Check sheet for the modelled part. Datum: model origin and axes. Units: mm. A direction names the side the tool comes from. Coordinates: 2 decimals unless noted, no trailing zeros. Loops run counter-clockwise (first coordinate to the right, second up) from the corner with the lowest first, then second, coordinate; pieces in that order, holes last. Notation, with made-up numbers: M -15,49.5 L 44,49.5 A31 ccw 44,84.5 Z; hole C -5,55.5 d3. An arc over 180 degrees is marked long. Return JSON: item names as keys, results as strings.
from build123d import *
from OCP.BRepAlgoAPI import BRepAlgoAPI_Cut
from OCP.TopTools import TopTools_ListOfShape

# Parameters (mm, degrees)
SKETCH1_W                = 20
SKETCH1_H                = 40
BOSS_EXTRUDE1_DEPTH      = 20
SKETCH3_W                = 18
SKETCH3_H                = 18
CUT_EXTRUDE1_DEPTH       = 20
BOSS_EXTRUDE2_START      = -1
BOSS_EXTRUDE2_DEPTH      = 1
BOSS_EXTRUDE3_START      = -1
SKETCH4_R                = 10
SKETCH4_R_2              = 5
BOSS_EXTRUDE3_DEPTH      = 1
SKETCH5_W                = 18
SKETCH5_H                = 18
CUT_EXTRUDE3_DEPTH       = 18
BOSS_EXTRUDE4_START      = -0.931933
SKETCH8_R                = 10
SKETCH8_R_2              = 5
BOSS_EXTRUDE4_DEPTH      = 0.931933
BOSS_EXTRUDE5_START      = -1.068067
BOSS_EXTRUDE5_DEPTH      = 1.068067
CUT_EXTRUDE4_OUTLINE_W   = 5
CUT_EXTRUDE4_OUTLINE_H   = 0.931933326
CUT_EXTRUDE4_OUTLINE_H_2 = 1.068066674
SKETCH12_R               = 5
CUT_EXTRUDE5_DEPTH       = 42.231056256


with BuildPart() as part:
    # Sketch1 → Boss-Extrude1 (new body)
    with BuildSketch(Plane(origin=(0, 0, 0), x_dir=(0, 0, -1), z_dir=(1, 0, 0))):
        Rectangle(SKETCH1_W, SKETCH1_H)
    extrude(amount=BOSS_EXTRUDE1_DEPTH)

    # Sketch3 → Cut-Extrude1 (cut)
    with BuildSketch(Plane.XZ.offset(20)):
        with Locations((9.965966663, 0)):
            Rectangle(SKETCH3_W, SKETCH3_H)
    extrude(amount=-CUT_EXTRUDE1_DEPTH, mode=Mode.SUBTRACT)

    # Sketch2 → Boss-Extrude2 (add)
    with BuildSketch(Plane.XY.offset(10).offset(BOSS_EXTRUDE2_START)):
        with BuildLine():
            ThreePointArc((0, -20), (10, -30), (20, -20))
            Line((20, -20), (0, -20))
        make_face()
    extrude(amount=BOSS_EXTRUDE2_DEPTH)

    # Sketch4 → Boss-Extrude3 (add)
    with BuildSketch(Plane(origin=(0, 0, -10), x_dir=(-1, 0, 0), z_dir=(0, 0, -1)).offset(BOSS_EXTRUDE3_START)):
        with Locations((-10, -20)):
            Circle(SKETCH4_R)
        with Locations((-10, -20)):
            Circle(SKETCH4_R_2, mode=Mode.SUBTRACT)
    extrude(amount=BOSS_EXTRUDE3_DEPTH)

    # Sketch5 → Cut-Extrude3 (cut)
    with BuildSketch(Plane(origin=(0, 20, 0), x_dir=(1, 0, 0), z_dir=(0, 1, 0))):
        with Locations((10.068066674, 0)):
            Rectangle(SKETCH5_W, SKETCH5_H)
    extrude(amount=-CUT_EXTRUDE3_DEPTH, mode=Mode.SUBTRACT)

    # Sketch8 → Boss-Extrude4 (add)
    with BuildSketch(Plane(origin=(20, 0, 0), x_dir=(0, 0, -1), z_dir=(1, 0, 0)).offset(BOSS_EXTRUDE4_START)):
        with Locations((0, 20)):
            Circle(SKETCH8_R)
        with Locations((0, 20)):
            Circle(SKETCH8_R_2, mode=Mode.SUBTRACT)
    extrude(amount=BOSS_EXTRUDE4_DEPTH)

    # Sketch7 → Boss-Extrude5 (add)
    with BuildSketch(Plane.ZY.offset(BOSS_EXTRUDE5_START)):
        with BuildLine():
            ThreePointArc((10, 20), (0, 30), (-10, 20))
            Line((-10, 20), (10, 20))
        make_face()
    extrude(amount=BOSS_EXTRUDE5_DEPTH)


with BuildPart() as cut_extrude4_tool:
    # Cut-Extrude4: read off the stored shape, not the designer's step
    # Cut-Extrude4 outline → Cut-Extrude4 (revolve)
    with BuildSketch(Plane(origin=(0, 20, 0), x_dir=(0, 1, 0), z_dir=(0, 0, -1))):
        with Locations((2.5, 19.534033337)):
            Rectangle(CUT_EXTRUDE4_OUTLINE_W, CUT_EXTRUDE4_OUTLINE_H)
        with Locations((2.5, 0.534033337)):
            Rectangle(CUT_EXTRUDE4_OUTLINE_W, CUT_EXTRUDE4_OUTLINE_H_2)
    revolve(axis=Axis((0, 20, 0), (1, 0, 0)))


with BuildPart() as part_1:
    add(part.part)

    # Cut-Extrude4: cut by cut_extrude4_tool, with a tolerance
    cut_extrude4_stock = TopTools_ListOfShape()
    cut_extrude4_stock.Append(part_1.part.wrapped)
    cut_extrude4_tools = TopTools_ListOfShape()
    cut_extrude4_tools.Append(cut_extrude4_tool.part.wrapped)
    cut_extrude4_cut = BRepAlgoAPI_Cut()
    cut_extrude4_cut.SetArguments(cut_extrude4_stock)
    cut_extrude4_cut.SetTools(cut_extrude4_tools)
    cut_extrude4_cut.SetFuzzyValue(0.00001)
    cut_extrude4_cut.Build()
    add(Compound.cast(cut_extrude4_cut.Shape()).solids(), mode=Mode.REPLACE)

    # Sketch12 → Cut-Extrude5 (cut, through all)
    with BuildSketch(Plane.XY.offset(10)):
        with Locations(Location((10, -20, 0), (0, 0, 90))):
            Circle(SKETCH12_R)
    extrude(amount=-CUT_EXTRUDE5_DEPTH, mode=Mode.SUBTRACT)


solid = part_1.part
1) Draft check along Y on faces 6 (the face through (10, 20, -9.5)), 7 (the face through (10, 11, -9)), 8 (the face through (9.78, -24.995, -9.493)). Enter one of: +Y half, -Y half, draft (parallel to the pull), parting line (faces both ways), or undercut.
Answers:
{"face 6": "+Y half", "face 7": "draft", "face 8": "undercut"}
2) Section check C-C on x = 3.75. Record the cut outline in (y, z), then the cut area to 3 significant figures.
Answers:
{"outline": "M -27.81,-10 L 20,-10 L 20,-9 L 2,-9 L 2,9 L 20,9 L 20,10 L -27.81,10 L -27.81,9 L 0,9 L 0,-9 L -27.81,-9 Z", "area": "132 mm²"}
3) Go/stop test with flat-tipped pins: pin 1 Ø9 at (x, z) = (12, -0.5) entering from -Y; pin 2 Ø0.8 at (x, z) = (19.5, 0.5) entering from -Y; pin 3 Ø2.5 at (x, z) = (12.5, 7.5) entering from +Y; pin 4 Ø2 at (y, z) = (21, -3.5) entering from +X. Record where each tip stops, or that it passes through.
Answers:
{"pin 1": "y = 0", "pin 2": "y = -20", "pin 3": "y = 2", "pin 4": "through"}
4) Section check D-D on z = -5.75. Record the cut outline in (x, y).
Answers:
{"outline": "M 0,-20 L 0.97,-20 L 0.97,0 L 18.97,0 L 18.97,-20 L 20,-20 L 20,28.18 L 19.07,28.18 L 19.07,2 L 1.07,2 L 1.07,28.18 L 0,28.18 Z"}
5) Section check B-B on z = 1. Record the cut outline in (x, y), then the cut area to 3 significant figures.
Answers:
{"outline": "M 0,-20 L 0.97,-20 L 0.97,0 L 18.97,0 L 18.97,-20 L 20,-20 L 20,15.1 L 19.07,15.1 L 19.07,2 L 1.07,2 L 1.07,15.1 L 0,15.1 Z; M 0,24.9 L 1.07,24.9 L 1.07,29.95 L 0,29.95 Z; M 19.07,24.9 L 20,24.9 L 20,29.95 L 19.07,29.95 Z", "area": "116 mm²"}
6) Set-up check for faces 1 (the face through (9.78, -24.995, 9.507)), 2 (the face through (19.068, 11, 0)), 3 (the face through (10, 20, 9.5)), 4 (the face through (10, 0, 0)), 5 (the face through (19.53, 15.12, 1.08)): record each of +Z, -Z, +X, -X, +Y, -Y from which the full face is reachable in a straight line by a thin tool's end or side.
Answers:
{"face 1": "+Z, -Z", "face 2": "+Y", "face 3": "+Z, -Z, +Y", "face 4": "-Y", "face 5": "+X, -X"}
7) Scan lines: line 1 along X through (y, z) = (27.5, 1.25); line 2 along X through (y, z) = (-5.5, -4.25); line 3 along Z through (x, y) = (14, 9). Record each from-to range of solid material in increasing order. Write a range as [from, to].
Answers:
{"line 1": "[0, 1.07], [19.07, 20]", "line 2": "[0, 0.97], [18.97, 20]", "line 3": "[-10, -9], [9, 10]"}
8) Section check A-A on x = 10. Record the cut outline in (y, z), then the cut area to 3 significant figures.
Answers:
{"outline": "M -30,-10 L -25,-10 L -25,-9 L -30,-9 Z; M -30,9 L -25,9 L -25,10 L -30,10 Z; M -15,-10 L 20,-10 L 20,-9 L 2,-9 L 2,9 L 20,9 L 20,10 L -15,10 L -15,9 L 0,9 L 0,-9 L -15,-9 Z", "area": "116 mm²"}
